The model under review builds one solid part; all positions refer to its coordinate system, in mm. Face numbers are marked on the shaded views. Round coordinates to 2 decimals unless told otherwise and drop trailing zeros. Write each loop counter-clockwise with the first axis right and the second up, starting at its lowest first coordinate (ties: lowest second). Pieces come first, ordered by that corner, then holes. Notation, with made-up numbers: (-2.75, 0) - (36.25, 0) arc R25 cw to (36.25, 20) - close; hole circle Ø5 at (84.25, 70.25). An arc over 180 degrees is marked (long way). One line per question, with ' | ' between items. Start each with the question number.
Solid Edge part; units mm, degrees
sketch "Sketch1" plane through (0, 0, 0) normal (0, 0, 1) x (1, 0, 0)
  line L0 (0, 0) -> (6.45, 0)
  line L1 (6.45, 0) -> (13.9141, -2)
  line L2 (13.9141, -2) -> (6.45, -4)
  line L3 (6.45, -4) -> (0, -4)
  line L4 (0, -4) -> (0, 0)
revolve "RevolvedProtrusion1" add sketch "Sketch1" angle 360 about axis through (0, -4, 0) along (0, 1, 0)
sketch "Sketch2" plane through (0, 0, 0) normal (0, -1, 0) x (1, 0, 0)
  line L0 (-26, -26) -> (-26, 26)
  line L1 (-26, 26) -> (26, 26)
  line L2 (26, 26) -> (26, -26)
  line L3 (26, -26) -> (-26, -26)
  line L4 (-6.5, 3.7528) -> (0, 7.5056)
  line L5 (0, 7.5056) -> (6.5, 3.7528)
  line L6 (6.5, 3.7528) -> (6.5, -3.7528)
  line L7 (6.5, -3.7528) -> (0, -7.5056)
  line L8 (0, -7.5056) -> (-6.5, -3.7528)
  line L9 (-6.5, -3.7528) -> (-6.5, 3.7528)
extrude "ExtrudedCutout_1" cut sketch "Sketch2" against normal blind 5 and the other way blind 5
sketch "Sketch3" plane through (0, 0, 0) normal (0, 0, 1) x (1, 0, 0)
  line L0 (0, 0) -> (4, 0)
  line L1 (4, 0) -> (3.3235, -0.6765)
  line L2 (3.3235, -0.6765) -> (3.3235, -3.3235)
  line L3 (3.3235, -3.3235) -> (4, -4)
  line L4 (4, -4) -> (0, -4)
  line L5 (0, -4) -> (0, 0)
revolve "RevolvedCutout1" cut sketch "Sketch3" angle 360 about axis through (0, -4, 0) along (0, 1, 0)
cosmetic_thread "Thread_1" thread depth 2.647
properties part number "DIN-439-B - M8(F)"
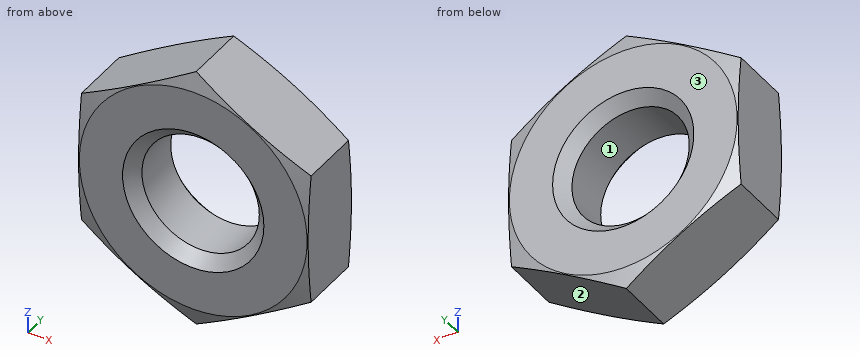
1. Add section A-A, the plane y = -0.85. Write out the cut boundary in (x, z), then the cut area to 3 significant figures.
2. The part is to be moulded in two halves that separate along X. For the marked faces 1, 2 and 3, say which applies: pulls with the +X half, pulls with the -X half, needs draft (parallel to the pull), parting line crosses it, or undercut.
3. Wall thickness on line 1 along X through (y, z) = (-2.8, 0); line 2 along Y through (x, z) = (-1.25, -3.5); line 3 along Z through (x, y) = (-3.25, -3.8): over which ranges is each line inside the solid? List them lowest first. Write a range as [from, to].
4. Add section B-B, the plane z = 0. Write out the cut boundary in (x, y).
5. Clearance check with a flat-ended pin moving along its axis: P1, Ø7.5, axis at x = 0, z = 0, coming from the +Y side. State where the tip first meets the part, or that it passes through.
Geometry check:
1) outline: (-6.5, -3.75) - (0, -7.51) - (6.5, -3.75) - (6.5, 3.75) - (0, 7.51) - (-6.5, 3.75) - close; hole circle Ø6.65 at (0, 0) | area: 112 mm2
2) face 1: undercut | face 2: pulls with the +X half | face 3: needs draft
3) line 1: x = [-6.5, -3.32], [3.32, 6.5] | line 2: y = [-3.72, -0.28] | line 3: z = [-5.63, -1.97], [1.97, 5.63]
4) outline: (-6.5, -3.99) - (-6.45, -4) - (-4, -4) - (-3.32, -3.32) - (-3.32, -0.68) - (-4, 0) - (-6.45, 0) - (-6.5, -0.01) - close; (3.32, -3.32) - (4, -4) - (6.45, -4) - (6.5, -3.99) - (6.5, -0.01) - (6.45, 0) - (4, 0) - (3.32, -0.68) - close
5) P1: stops at y = -0.25
